Part model, mm, in its own coordinate system. Round coordinates to 2 decimals unless told otherwise and drop trailing zeros. Order: outer loops, then holes, each group sorted by start corner. A loop starts at its lowest first (then second) coordinate and runs counter-clockwise, first axis right, second up. Notation, with made-up numbers: (19.25, -23) - (72.25, -23) arc R18 ccw to (72.25, -7) - close; hole circle Ø6 at (57.25, -25.75). An arc over 180 degrees is marked (long way). Answer as a JSON object with one key per item and string values.
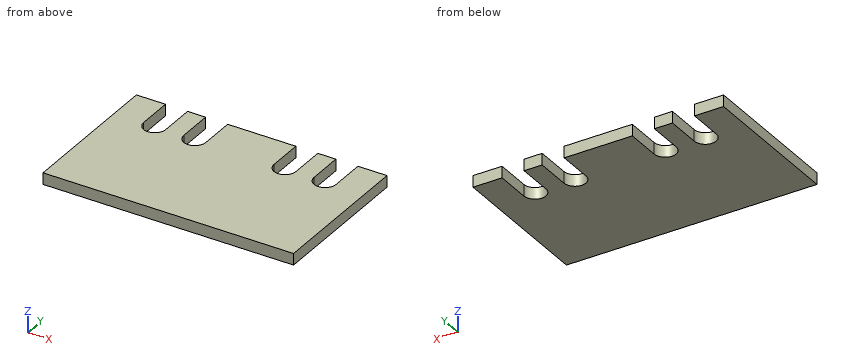
```python
from build123d import *

# Parameters (mm, degrees)
PAD_DEPTH = 2.3


with BuildPart() as part:
    # Sketch → Pad (new body)
    with BuildSketch(Plane.XY):
        with BuildLine():
            Line((0, 0), (50, 0))
            Line((50, 0), (50, 30))
            Line((44.2, 30), (50, 30))
            Line((44.2, 30), (44.2, 23))
            ThreePointArc((39.8, 23), (42, 20.8), (44.2, 23))
            Line((39.8, 23), (39.8, 30))
            Line((39.8, 30), (36.2, 30))
            Line((36.2, 30), (36.2, 23))
            ThreePointArc((31.8, 23), (34, 20.8), (36.2, 23))
            Line((31.8, 23), (31.8, 30))
            Line((31.8, 30), (18.2, 30))
            Line((18.2, 30), (18.2, 23))
            ThreePointArc((13.8, 23), (16, 20.8), (18.2, 23))
            Line((13.8, 23), (13.8, 30))
            Line((13.8, 30), (10.2, 30))
            Line((10.2, 30), (10.2, 23))
            ThreePointArc((5.8, 23), (8, 20.8), (10.2, 23))
            Line((5.8, 23), (5.8, 30))
            Line((5.8, 30), (0, 30))
            Line((0, 30), (0, 0))
        make_face()
    extrude(amount=PAD_DEPTH)


solid = part.part
```
Item 1: Cut at C-C (x = 32.5). Write the cut outline in (y, z).
Taken from the geometry:
{"outline": "(0, 0) - (21.39, 0) - (21.39, 2.3) - (0, 2.3) - close"}
Item 2: Cut at B-B (x = 42). Write the cut outline in (y, z).
Taken from the geometry:
{"outline": "(0, 0) - (20.8, 0) - (20.8, 2.3) - (0, 2.3) - close"}
Item 3: Cut at A-A (z = 1.1). Write the cut outline in (x, y).
Taken from the geometry:
{"outline": "(0, 0) - (50, 0) - (50, 30) - (44.2, 30) - (44.2, 23) arc R2.2 cw to (39.8, 23) - (39.8, 30) - (36.2, 30) - (36.2, 23) arc R2.2 cw to (31.8, 23) - (31.8, 30) - (18.2, 30) - (18.2, 23) arc R2.2 cw to (13.8, 23) - (13.8, 30) - (10.2, 30) - (10.2, 23) arc R2.2 cw to (5.8, 23) - (5.8, 30) - (0, 30) - close"}
Item 4: Drop a flat-ended pin along its axis: P1, Ø12, axis at x = 12.5, y = 3, coming from the -Z side. Give the stop position or say it passes through.
Taken from the geometry:
{"P1": "z = 0"}
Item 5: Probe L1, parallel to X at y = 23, z = 1.25; L2, parallel to X at y = 21, z = 1.8; L3, parallel to Y at x = 8, z = 2.2. List the from-to ranges inside material, lowest first. Write a range as from..to.
Taken from the geometry:
{"L1": "0..5.8, 10.2..13.8, 18.2..31.8, 36.2..39.8, 44.2..50", "L2": "0..7.08, 8.92..15.08, 16.92..33.08, 34.92..41.08, 42.92..50", "L3": "0..20.8"}
